Read the model definition and answer for the solid it produces. Units are mm, in the model's axes. Face numbers are marked on the shaded views. A direction names the side the tool comes from. Give positions to 0.01 mm unless a question says otherwise; leave off trailing zeros. Loops run counter-clockwise (first coordinate to the right, second up) from the corner with the lowest first, then second, coordinate; pieces in that order, holes last. Notation, with made-up numbers: (13, 32.5) - (67, 32.5) arc R20 cw to (67, 69.5) - close; hole circle Ø9 at (67.25, -18.75). An arc over 180 degrees is marked (long way). Use a Markdown table: item, result. Add a question column.
Item 1: A cutting plane is placed at C-C (z = 0). Determine the outline of the cut face in (x, y), plus the area to 3 significant figures.
Item 2: Each of these flat-tipped pins is pushed along its axis until it touches: P1, Ø1.5, axis at y = 2, z = -3, coming from the -X side; P2, Ø1.5, axis at x = -2.5, y = 1.5, coming from the -Z side; P3, Ø1.5, axis at x = 1, z = 4, coming from the +Y side. Where does it stop, or does it pass through?
Item 3: Which of the six approach directions +Z, -Z, +X, -X, +Y, -Y give full straight-line access (tool end or side, diameter ignored) to the marked faces 1, 2, 3, 4 and 5?
Item 4: A cutting plane is placed at A-A (x = -2). Determine the outline of the cut face in (y, z), plus the area to 3 significant figures.
Item 5: A cutting plane is placed at B-B (y = 1.25). Determine the outline of the cut face in (x, z).
Item 6: Consider probe 1 along X at (y, z) = (3, 1.5); probe 2 along X at (y, z) = (4.25, -3.5). Determine where each line is inside the solid, lowest interval first. Write a range as [from, to].
Item 7: A cutting plane is placed at D-D (y = 3). Determine the outline of the cut face in (x, z), plus the area to 3 significant figures.
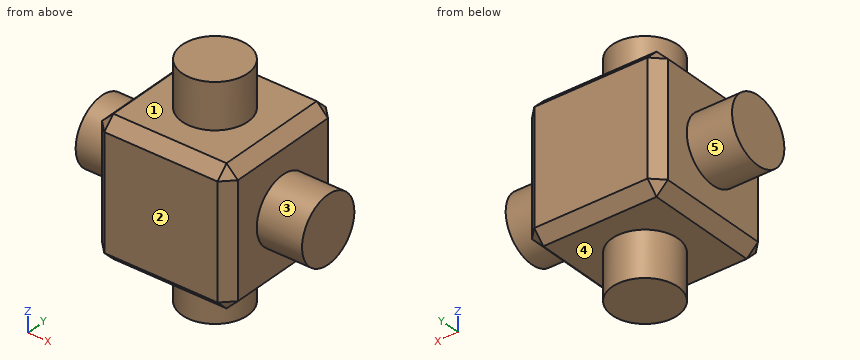
from build123d import *

# Parameters (mm, degrees)
SKETCH1_W                = 6
SKETCH1_H                = 6
BOSS_EXTRUDE1_DEPTH      = 6
SKETCH2_R                = 1.45
BOSS_EXTRUDE2_DEPTH      = 2
BOSS_EXTRUDE2_DEPTH_BACK = 8
SKETCH3_R                = 1.45
BOSS_EXTRUDE3_DEPTH      = 2
BOSS_EXTRUDE3_DEPTH_BACK = 8
CHAMFER1_SIZE            = 0.5


with BuildPart() as part:
    # Sketch1 → Boss-Extrude1 (new body)
    with BuildSketch(Plane(origin=(0, 0, 0), x_dir=(1, 0, 0), z_dir=(0, 1, 0))):
        Rectangle(SKETCH1_W, SKETCH1_H)
    extrude(amount=BOSS_EXTRUDE1_DEPTH)

    # Sketch2 → Boss-Extrude2 (add, two sides)
    with BuildSketch(Plane(origin=(3, 0, 0), x_dir=(0, 0, -1), z_dir=(1, 0, 0))) as boss_extrude2_sk:
        with Locations((0, 3)):
            Circle(SKETCH2_R)
    extrude(amount=BOSS_EXTRUDE2_DEPTH)
    extrude(boss_extrude2_sk.sketch, amount=-BOSS_EXTRUDE2_DEPTH_BACK)

    # Sketch3 → Boss-Extrude3 (add, two sides)
    with BuildSketch(Plane.XY.offset(3)) as boss_extrude3_sk:
        with Locations((0, 3)):
            Circle(SKETCH3_R)
    extrude(amount=BOSS_EXTRUDE3_DEPTH)
    extrude(boss_extrude3_sk.sketch, amount=-BOSS_EXTRUDE3_DEPTH_BACK)

    # Chamfer1
    chamfer1_edges = [part.edges().sort_by_distance(p)[0] for p in [
        (-3, 6, 0),
        (0, 6, 3),
        (3, 6, 0),
        (0, 0, 3),
        (-3, 0, 0),
        (0, 0, -3),
        (3, 0, 0),
        (3, 3, 3),
        (-3, 3, 3),
        (-3, 3, -3),
        (3, 3, -3),
        (0, 6, -3),
    ]]
    chamfer(chamfer1_edges, length=CHAMFER1_SIZE)


solid = part.part
Geometry says:
| question | item | result |
|---|---|---|
| 1 | outline | (-5, 1.55) - (-3, 1.55) - (-3, 0.5) - (-2.5, 0) - (2.5, 0) - (3, 0.5) - (3, 1.55) - (5, 1.55) - (5, 4.45) - (3, 4.45) - (3, 5.5) - (2.5, 6) - (-2.5, 6) - (-3, 5.5) - (-3, 4.45) - (-5, 4.45) - close |
| 1 | area | 47.1 mm² |
| 2 | P1 | x = -3 |
| 2 | P2 | z = -3 |
| 2 | P3 | y = 4.43 |
| 3 | face 1 | +Z |
| 3 | face 2 | +Z, -Z, +X, -X, -Y |
| 3 | face 3 | +X |
| 3 | face 4 | -Z |
| 3 | face 5 | -X |
| 4 | outline | (0, -2.5) - (0.5, -3) - (5.5, -3) - (6, -2.5) - (6, 2.5) - (5.5, 3) - (0.5, 3) - (0, 2.5) - close |
| 4 | area | 35.5 mm² |
| 5 | outline | (-3, -2.5) - (-2.5, -3) - (2.5, -3) - (3, -2.5) - (3, 2.5) - (2.5, 3) - (-2.5, 3) - (-3, 2.5) - close |
| 6 | probe 1 | [-3, 3] |
| 6 | probe 2 | [-0.73, 0.73] |
| 7 | outline | (-5, -1.45) - (-3, -1.45) - (-3, -2.5) - (-2.5, -3) - (-1.45, -3) - (-1.45, -5) - (1.45, -5) - (1.45, -3) - (2.5, -3) - (3, -2.5) - (3, -1.45) - (5, -1.45) - (5, 1.45) - (3, 1.45) - (3, 2.5) - (2.5, 3) - (1.45, 3) - (1.45, 5) - (-1.45, 5) - (-1.45, 3) - (-2.5, 3) - (-3, 2.5) - (-3, 1.45) - (-5, 1.45) - close |
| 7 | area | 58.7 mm² |
